Read the model definition and answer for the solid it produces. Units are mm, in the model's axes. A direction names the side the tool comes from. Coordinates: 2 decimals unless noted, no trailing zeros. Order: outer loops, then holes, each group sorted by start corner. A loop starts at its lowest first (then second) coordinate and runs counter-clockwise, first axis right, second up. Notation, with made-up numbers: (84.25, 44) -> (120.25, 44) arc R15 ccw to (120.25, 48) -> close; hole circle Ø9 at (26.25, -32.75). An arc over 180 degrees is marked (long way). Answer as a JSON object with one key per item and string values. Group by question number.
1) Given pin 1 (2 mm diameter, centred on y = 4, z = -6.5, fed in from -X); pin 2 (2.5 mm diameter, centred on x = 0, z = -6, fed in from -Y); pin 3 (2 mm diameter, centred on x = 17.5, z = -9, fed in from -Y); pin 4 (3.5 mm diameter, centred on x = 0, z = 0, fed in from -Y), each flat-ended and moving along its own axis, determine where each tip first touches the part or whether it passes through.
2) Section B-B on z = -6 is taken. Determine the outline of the cut face in (x, y), and give its area (3 significant figures).
3) Section C-C on z = 0 is taken. Determine the outline of the cut face in (x, y), and give its area (3 significant figures).
4) Determine the mould class of faces 3 (the cylindrical face through (0.325, 5.916, 7.464)), 4 (the cylindrical face through (29.97, 5.92, -1.32)), 5 (the flat face through (0, 12, 0)) for opening direction Z: released by +Z, released by -Z, zero draft, split by the parting line, or undercut.
5) Section D-D on y = 9.5 is taken. Determine the outline of the cut face in (x, z), and give its area (3 significant figures).
6) A tool of negligible diameter and unlimited length cuts with its end or side. For faces 1 (the flat face through (-6, 0, 0)), 2 (the flat face through (0, 3, 0)), from which of +Z, -Z, +X, -X, +Y, -Y can it reach the whole face along a straight path? Write none if from no direction.
7) Section A-A on x = 0 is taken. Determine the outline of the cut face in (y, z).
8) Consider L1, parallel to Z at x = 0, y = 7.75; L2, parallel to Z at x = 0, y = 2.75; L3, parallel to X at y = 3.75, z = -6.5. Determine where each line is inside the solid, lowest interval first.
Autodesk Inventor part; units mm, degrees
ref_plane "YZ Plane" through (0, 0, 0) normal (1, 0, 0) x (0, 1, 0)
ref_plane "XZ Plane" through (0, 0, 0) normal (0, 1, 0) x (-1, 0, 0)
ref_plane "XY Plane" through (0, 0, 0) normal (0, 0, 1) x (1, 0, 0)
sketch "スケッチ1" plane through (0, 0, 0) normal (0, 1, 0) x (-1, 0, 0)
  circle A0 centre (0, 0) radius 30
  circle A1 centre (0, 6) radius 1.5
  circle A2 centre (0, -6) radius 1.5
  circle A3 centre (0, 0) radius 3
  dimension "d0" = 60
  dimension "d1" = 9
  dimension "d2" = 6
  dimension "d3" = 3
  dimension "d4" = 3
  dimension "d5" = 6
  dimension "d6" = 6
extrude "押し出し1" add sketch "スケッチ1" along normal blind 12 contours A0 | A3
extrude "押し出し2" cut sketch "スケッチ1" along normal blind 3 contours A3
properties part number "タイヤ" material "木材 (オーク)"
Worked answers:
{
 "1": {"pin 1": "stops at x = -29.49", "pin 2": "passes through", "pin 3": "stops at y = 0", "pin 4": "stops at y = 3"},
 "2": {"outline": "(-29.39, 0) -> (-1.5, 0) -> (-1.5, 12) -> (-29.39, 12) -> close; (1.5, 0) -> (29.39, 0) -> (29.39, 12) -> (1.5, 12) -> close", "area": "669 mm²"},
 "3": {"outline": "(-30, 0) -> (-3, 0) -> (-3, 3) -> (3, 3) -> (3, 0) -> (30, 0) -> (30, 12) -> (-30, 12) -> close", "area": "702 mm²"},
 "4": {"face 3": "undercut", "face 4": "split by the parting line", "face 5": "zero draft"},
 "5": {"outline": "circle Ø60 at (0, 0); hole circle Ø3 at (0, -6); hole circle Ø3 at (0, 6)", "area": "2,810 mm²"},
 "6": {"face 1": "+Z, -Z, +X, -X, -Y", "face 2": "-Y"},
 "7": {"outline": "(0, -30) -> (12, -30) -> (12, -7.5) -> (0, -7.5) -> close; (0, -4.5) -> (12, -4.5) -> (12, 4.5) -> (0, 4.5) -> (0, 3) -> (3, 3) -> (3, -3) -> (0, -3) -> close; (0, 7.5) -> (12, 7.5) -> (12, 30) -> (0, 30) -> close"},
 "8": {"L1": "z = -30 to -7.5, -4.5 to 4.5, 7.5 to 30", "L2": "z = -30 to -7.5, -4.5 to -3, 3 to 4.5, 7.5 to 30", "L3": "x = -29.29 to -1.41, 1.41 to 29.29"}
}
